```python
from build123d import *

# Parameters (mm, degrees)
ATTACHMENTBOLTHOLES_START = -4
SKETCH11_R                = 1.325
ATTACHMENTBOLTHOLES_DEPTH = 19.6
SKETCH13_R                = 1.975
SHAFTBOLTHEAD_DEPTH       = 2.2
SHAFTBOLTTHRU_START       = -4
SKETCH14_R                = 1.1
SHAFTBOLTTHRU_DEPTH       = 19.6
NUTHOLE_DEPTH             = 12.6
CIRPATTERN1_COUNT         = 4


with BuildPart() as part:
    # Sketch10 → Revolve1 (revolve)
    with BuildSketch(Plane(origin=(0, 0, 0), x_dir=(1, 0, 0), z_dir=(0, 1, 0))):
        Polygon((-13.45, 3), (-7.5, 3), (-7.5, 2), (-5, 2), (-5, -14.6), (-12.5, -14.6), (-12.5, 0), (-13.45, 0), align=None)
    revolve(axis=Axis((0, 0, -38.468953364), (0, 0, 1)))

    # Sketch11 → AttachmentBoltHoles (cut)
    with BuildSketch(Plane.XY.offset(ATTACHMENTBOLTHOLES_START)):
        with Locations((9.5, 0)):
            Circle(SKETCH11_R)
    attachmentboltholes = extrude(amount=ATTACHMENTBOLTHOLES_DEPTH, mode=Mode.SUBTRACT)

    # Sketch13 → ShaftBoltHead (cut)
    with BuildSketch(Plane(origin=(0, 0, -3), x_dir=(-1, 0, 0), z_dir=(0, 0, -1))):
        with Locations((-7.071067812, 7.071067812)):
            Circle(SKETCH13_R)
    shaftbolthead = extrude(amount=-SHAFTBOLTHEAD_DEPTH, mode=Mode.SUBTRACT)

    # Sketch14 → ShaftBoltThru (cut)
    with BuildSketch(Plane.XY.offset(SHAFTBOLTTHRU_START)):
        with Locations((7.071067812, 7.071067812)):
            Circle(SKETCH14_R)
    shaftboltthru = extrude(amount=SHAFTBOLTTHRU_DEPTH, mode=Mode.SUBTRACT)

    # Sketch12 → NutHole (cut)
    with BuildSketch(Plane.XY.offset(14.6)):
        Polygon((12.075, -1.486676943), (12.075, 1.486676943), (9.5, 2.973353886), (6.925, 1.486676943), (6.925, -1.486676943), (9.5, -2.973353886), align=None)
    nuthole = extrude(amount=-NUTHOLE_DEPTH, mode=Mode.SUBTRACT)

    # CirPattern1: AttachmentBoltHoles, ShaftBoltHead, ShaftBoltThru, NutHole ×4 about axis
    cirpattern1_axis = Axis((0, 0, 0), (0, 0, 1))
    for i in range(1, CIRPATTERN1_COUNT):
        add(attachmentboltholes.rotate(cirpattern1_axis, i * 360 / CIRPATTERN1_COUNT), mode=Mode.SUBTRACT)
        add(shaftbolthead.rotate(cirpattern1_axis, i * 360 / CIRPATTERN1_COUNT), mode=Mode.SUBTRACT)
        add(shaftboltthru.rotate(cirpattern1_axis, i * 360 / CIRPATTERN1_COUNT), mode=Mode.SUBTRACT)
        add(nuthole.rotate(cirpattern1_axis, i * 360 / CIRPATTERN1_COUNT), mode=Mode.SUBTRACT)


solid = part.part
```
Work out the finished part from the listing and answer in its coordinate system (mm). A direction names the side the tool comes from. Coordinates: 2 decimals unless noted, no trailing zeros. Write each loop counter-clockwise with the first axis right and the second up, starting at its lowest first coordinate (ties: lowest second). Pieces come first, ordered by that corner, then holes.
Q1. A cutting plane is placed at B-B, the plane y = -6.5. Give the vertices of the cut face in (x, z).
Q2. A cutting plane is placed at A-A, the plane x = 0. State how many separate pieces and enclosed holes the cut face has, then the cut area to 3 significant figures.
Q3. Which of the six approach directions +Z, -Z, +X, -X, +Y, -Y give full straight-line access (tool end or side, diameter ignored) to faces 4 (the face through (-0.398, 10.764, -0.535)), 5 (the face through (7.493, -0.33, -2.493)), 6 (the face through (6.925, 0, 8))?
Q4. Each of these flat-tipped pins is pushed along its axis until it touches: pin 1 Ø5 at (y, z) = (-3.5, -1) entering from -X; pin 2 Ø1.5 at (x, z) = (3.5, 6) entering from +Y; pin 3 Ø1.5 at (x, z) = (0, 10.5) entering from -Y. Where does it stop, or does it pass through?
Q5. A cutting plane is placed at D-D, the plane x = -4. Give the vertices of the cut face in (y, z), then the cut area to 3 significant figures.
Q6. Determine the mould class of faces 1 (the face through (-11.923, -3.755, 7.198)), 2 (the face through (2.22, 8.194, 8.388)), 3 (the face through (-0.2, 5.4, 14.6)) for opening direction X: released by +X, released by -X, zero draft, split by the parting line, or undercut.
Q7. Find the intervals of material crossed by line 1 (Y direction, x = 0.25, z = 6.5) (1 decimal); line 2 (X direction, y = 1.25, z = 5.5) (3 decimals); line 3 (X direction, y = 0.75, z = 12.75) (3 decimals), in increasing order.
Findings below:
1. outline: (-11.78, -3) - (-8.96, -3) - (-8.96, -0.8) - (-8.01, -0.8) - (-8.01, 14.6) - (-10.68, 14.6) - (-10.68, 0) - (-11.78, 0) - close; (-6.13, -0.8) - (-5.18, -0.8) - (-5.18, -3) - (-3.74, -3) - (-3.74, -2) - (3.74, -2) - (3.74, -3) - (5.18, -3) - (5.18, -0.8) - (6.13, -0.8) - (6.13, 14.6) - (-6.13, 14.6) - close; (8.01, -0.8) - (8.96, -0.8) - (8.96, -3) - (11.78, -3) - (11.78, 0) - (10.68, 0) - (10.68, 14.6) - (8.01, 14.6) - close
2. separate pieces: 4
2. enclosed holes: 0
2. area: 108 mm2
3. face 4: +Z, -Z
3. face 5: -Z
3. face 6: +Z
4. pin 1: stops at x = -13.41
4. pin 2: stops at y = 12.19
4. pin 3: stops at y = -12.5
5. outline: (-12.84, -3) - (-6.34, -3) - (-6.34, -2) - (-3, -2) - (-3, 14.6) - (-11.84, 14.6) - (-11.84, 0) - (-12.84, 0) - close; (3, -2) - (6.34, -2) - (6.34, -3) - (12.84, -3) - (12.84, 0) - (11.84, 0) - (11.84, 14.6) - (3, 14.6) - close
5. area: 311 mm2
6. face 1: split by the parting line
6. face 2: undercut
6. face 3: zero draft
7. line 1: y = -12.5 to -12.1, -6.9 to -5, 5 to 6.9, 12.1 to 12.5
7. line 2: x = -12.437 to -12.075, -6.925 to -4.841, 4.841 to 6.925, 12.075 to 12.437
7. line 3: x = -12.477 to -12.075, -6.925 to -4.943, 4.943 to 6.925, 12.075 to 12.477
